from build123d import *

# Parameters (mm, degrees)
SKETCH_1_R      = 100
EXTRUDE_1_DEPTH = 10
EXTRUDE_2_DEPTH = 20
CHAMFER_1_SIZE  = 2
CHAMFER_2_SIZE  = 2


with BuildPart() as part:
    # 草图1 → 凸台-拉伸1 (new body)
    with BuildSketch(Plane(origin=(0, 0, 0), x_dir=(1, 0, 0), z_dir=(0, 1, 0))):
        with Locations(Location((0, 0, 0), (0, 0, 270))):
            Circle(SKETCH_1_R)
    extrude(amount=EXTRUDE_1_DEPTH)

    # 草图2 → 凸台-拉伸2 (add, symmetric)
    with BuildSketch(Plane.XY):
        with BuildLine():
            Line((51.398957954, 25), (51.398957954, 10))
            Line((51.398957954, 10), (76.398957954, 10))
            Line((76.398957954, 10), (76.398957954, 25))
            ThreePointArc((76.398957954, 25), (63.898957954, 37.5), (51.398957954, 25))
        make_face()
    extrude(amount=EXTRUDE_2_DEPTH, both=True)

    # 倒角1
    chamfer_1_edges = [part.edges().sort_by_distance(p)[0] for p in [
        (51.398957954, 17.5, 20),
        (76.398957954, 17.5, 20),
        (63.898957954, 37.5, -20),
        (51.398957954, 17.5, -20),
        (76.398957954, 17.5, -20),
        (63.898957954, 37.5, 20),
    ]]
    chamfer(chamfer_1_edges, length=CHAMFER_1_SIZE)

    # 倒角2
    chamfer_2_edges = [part.edges().sort_by_distance(p)[0] for p in [
        (0, 10, -100),
    ]]
    chamfer(chamfer_2_edges, length=CHAMFER_2_SIZE)


solid = part.part
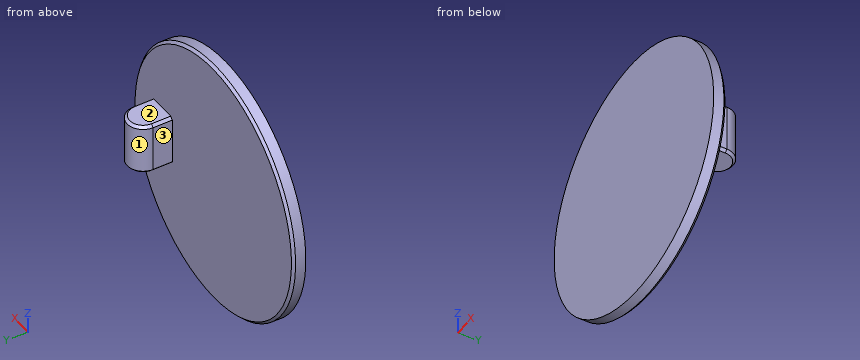
The listing builds one solid part. Answer for the finished solid, in the listing's coordinates (mm). Face numbers are marked on the shaded views. A direction names the side the tool comes from. Round coordinates to 2 decimals unless told otherwise and drop trailing zeros. Order: outer loops, then holes, each group sorted by start corner. A loop starts at its lowest first (then second) coordinate and runs counter-clockwise, first axis right, second up. Notation, with made-up numbers: M -21.5,21 L 36.5,21 A10 ccw 36.5,29 Z; hole C 18,-37.75 d7. An arc over 180 degrees is marked long. Answer in a Markdown table with one row per item. Add a question column.
1) The part is cut by section B-B on z = 0. Determine the outline of the cut face in (x, y), plus the area to 3 significant figures.
2) Which of the six approach directions +Z, -Z, +X, -X, +Y, -Y give full straight-line access (tool end or side, diameter ignored) to the marked faces 1, 2 and 3?
3) Consider line 1 along Z through (x, y) = (56.5, 19); line 2 along Y through (x, z) = (-45.5, 89); line 3 along Y through (x, z) = (-83, 2.5). Determine where each line is inside the solid, lowest interval first. Write a range as from..to.
4) Flat-ended cylindrical pins translate along their axes: pin 1 Ø12 at (y, z) = (21, -8.5) entering from -X; pin 2 Ø1 at (x, z) = (53, 77) entering from +Y; pin 3 Ø6 at (y, z) = (7.5, -7.5) entering from +X. Find the tip coordinate at first contact, or state that the pin passes through.
5) The part is cut by section A-A on x = 0. Determine the outline of the cut face in (y, z).
Findings below:
| question | item | result |
|---|---|---|
| 1 | outline | M -100,0 L 100,0 L 100,8 L 98,10 L 76.4,10 L 76.4,25 A12.5 ccw 51.4,25 L 51.4,10 L -98,10 L -100,8 Z |
| 1 | area | 2,620 mm² |
| 2 | face 1 | +Z, -Z, +Y |
| 2 | face 2 | +Z, +X, -X, +Y |
| 2 | face 3 | +Z, -Z, -X, +Y |
| 3 | line 1 | z = -20..20 |
| 3 | line 2 | y = 0..8.04 |
| 3 | line 3 | y = 0..10 |
| 4 | pin 1 | stops at x = 51.4 |
| 4 | pin 2 | stops at y = 10 |
| 4 | pin 3 | stops at x = 99.9 |
| 5 | outline | M 0,-100 L 8,-100 L 10,-98 L 10,98 L 8,100 L 0,100 Z |
